```python
from build123d import *

# Parameters (mm, degrees)
SKETCH_1_W                  = 25
SKETCH_1_H                  = 62
EXTRUDE_1_DEPTH             = 10
PATTERN_LINEAR_1_COUNT      = 2
PATTERN_LINEAR_1_PITCH      = 16
PATTERN_LINEAR_1_COUNT_DIR2 = 2
PATTERN_LINEAR_1_PITCH_DIR2 = 52


with BuildPart() as part:
    # Sketch 1 → Extrude 1 (new body)
    with BuildSketch(Plane(origin=(0, 0, 0), x_dir=(0, 0, -1), z_dir=(1, 0, 0))):
        Rectangle(SKETCH_1_W, SKETCH_1_H)
    extrude(amount=EXTRUDE_1_DEPTH)

    # Sketch 2 → Cut-Revolve 1 (revolve, cut)
    with BuildSketch(Plane(origin=(0, 26, 0), x_dir=(1, 0, 0), z_dir=(0, 1, 0)), mode=Mode.PRIVATE) as cut_revolve_1_sk:
        Polygon((0, 8), (0, 10.5), (0.433, 10.067), (9.567, 10.067), (10, 10.5), (10, 8), align=None)
    cut_revolve_1 = revolve(cut_revolve_1_sk.sketch.rotate(Axis((10, 26, -8), (-1, 0, 0)), 180), axis=Axis((10, 26, -8), (-1, 0, 0)), mode=Mode.SUBTRACT)

    # Pattern Linear 1: Cut-Revolve 1 2 × 2
    with Locations(*[(0, -j * PATTERN_LINEAR_1_PITCH_DIR2, i * PATTERN_LINEAR_1_PITCH) for i in range(PATTERN_LINEAR_1_COUNT) for j in range(PATTERN_LINEAR_1_COUNT_DIR2) if (i, j) != (0, 0)]):
        add(cut_revolve_1, mode=Mode.SUBTRACT)

    # Sketch 4 → Cut-Revolve 2 (revolve, cut)
    with BuildSketch(Plane(origin=(0, 23, 0), x_dir=(1, 0, 0), z_dir=(0, 1, 0)), mode=Mode.PRIVATE) as cut_revolve_2_sk:
        Polygon((0, 0), (0, 3.8), (5.555555556, 3.8), (5.555555556, 3.5), (2.055555556, 3.5), (1.555555556, 3), (1.555555556, 1.5), (4.155555556, 1.5), (5.021580959, 0), align=None)
    revolve(cut_revolve_2_sk.sketch.rotate(Axis((5.021580959, 23, 0), (-1, 0, 0)), 180), axis=Axis((5.021580959, 23, 0), (-1, 0, 0)), mode=Mode.SUBTRACT)

    # Sketch 5 → Cut-Revolve 3 (revolve, cut)
    with BuildSketch(Plane(origin=(0, 0, 0), x_dir=(1, 0, 0), z_dir=(0, 1, 0)), mode=Mode.PRIVATE) as cut_revolve_3_sk:
        Polygon((0, 0), (0, 3.8), (5.555555556, 3.8), (5.555555556, 3.5), (2.055555556, 3.5), (1.555555556, 3), (1.555555556, 1.5), (4.155555556, 1.5), (5.021580959, 0), align=None)
    revolve(cut_revolve_3_sk.sketch.rotate(Axis((5.021580959, 0, 0), (-1, 0, 0)), 180), axis=Axis((5.021580959, 0, 0), (-1, 0, 0)), mode=Mode.SUBTRACT)

    # Sketch 6 → Cut-Revolve 4 (revolve, cut)
    with BuildSketch(Plane(origin=(0, -23, 0), x_dir=(1, 0, 0), z_dir=(0, 1, 0)), mode=Mode.PRIVATE) as cut_revolve_4_sk:
        Polygon((0, 0), (0, 3.8), (5.555555556, 3.8), (5.555555556, 3.5), (2.055555556, 3.5), (1.555555556, 3), (1.555555556, 1.5), (4.155555556, 1.5), (5.021580959, 0), align=None)
    revolve(cut_revolve_4_sk.sketch.rotate(Axis((5.021580959, -23, 0), (-1, 0, 0)), 180), axis=Axis((5.021580959, -23, 0), (-1, 0, 0)), mode=Mode.SUBTRACT)

    # Sketch 7 → Revolve 1 (revolve)
    with BuildSketch(Plane(origin=(0, 0, 0), x_dir=(1, 0, 0), z_dir=(0, 1, 0)), mode=Mode.PRIVATE) as revolve_1_sk:
        Polygon((10, 0), (10, 4), (21.6, 4), (22, 3.6), (22, 0), align=None)
    revolve(revolve_1_sk.sketch.rotate(Axis((22, 0, 0), (-1, 0, 0)), 180), axis=Axis((22, 0, 0), (-1, 0, 0)))

    # Sketch 8 → Revolve 2 (revolve)
    with BuildSketch(Plane(origin=(0, -23, 0), x_dir=(1, 0, 0), z_dir=(0, 1, 0)), mode=Mode.PRIVATE) as revolve_2_sk:
        Polygon((10, 0), (10, 5), (52.6, 5), (53, 4.6), (53, 0), align=None)
    revolve(revolve_2_sk.sketch.rotate(Axis((53, -23, 0), (-1, 0, 0)), 180), axis=Axis((53, -23, 0), (-1, 0, 0)))

    # Sketch 9 → Revolve 3 (revolve)
    with BuildSketch(Plane(origin=(0, 23, 0), x_dir=(1, 0, 0), z_dir=(0, 1, 0)), mode=Mode.PRIVATE) as revolve_3_sk:
        Polygon((10, 0), (10, 5), (52.6, 5), (53, 4.6), (53, 0), align=None)
    revolve(revolve_3_sk.sketch.rotate(Axis((53, 23, 0), (-1, 0, 0)), 180), axis=Axis((53, 23, 0), (-1, 0, 0)))


solid = part.part
```
Can you work these out from the model? Positions are in its coordinate system, mm. A direction names the side the tool comes from. Give positions to 0.01 mm unless a question says otherwise; leave off trailing zeros. Order: outer loops, then holes, each group sorted by start corner. A loop starts at its lowest first (then second) coordinate and runs counter-clockwise, first axis right, second up. Notation, with made-up numbers: (66.5, -36.75) - (78.5, -36.75) arc R22 ccw to (78.5, -13.75) - close; hole circle Ø3 at (33, 79.5). An arc over 180 degrees is marked (long way). Use a Markdown table: item, result. Add a question column.
Q1. If we section it at D-D on z = -7.75: Count the separate pieces of the cut face and the enclosed holes in it, plus the area to 3 significant figures.
Q2. Please list where these lines run through material, in increasing order: line 1 along Y through (x, z) = (12.5, 3.25); line 2 along Y through (x, z) = (1.1, 0); line 3 along Y through (x, z) = (18.5, 1.75).
Q3. On a 3-axis mill with a long thin cutter (end or side, diameter ignored), from which of +Z, -Z, +X, -X, +Y, -Y can I reach the whole of each face in a straight line? I mean faces 1 (the flat face through (53, 23, 0)), 2 (the flat face through (1.556, -24.3, 1.3)). Say none if no direction works.
Q4. If we section it at B-B on x = 28: Write out the boundary of the cut face in (y, z), plus the area to 3 significant figures.
Q5. If we section it at C-C on y = 15.5: Write out the boundary of the cut face in (x, z).
Q6. I'm going to push flat-ended pins straight in: pin 1 (3 mm diameter, centred on y = 24.5, z = 1, fed in from -X); pin 2 (6 mm diameter, centred on x = 18, y = 5, fed in from +Z); pin 3 (3 mm diameter, centred on y = -5, z = -4, fed in from +X). Where does each tip first touch, or does it pass through?
Q7. If we mould it in two halves opening along Y, with no side actions, what happens to faces 3 (the flat face through (53, -23, 0)), 4 (the flat face through (10, 0, 6))? For each: released by +Y, released by -Y, zero draft, split by the parting line, or undercut.
Q8. If we section it at A-A on z = 8: Write out the boundary of the cut face in (x, y).
Answers follow:
| question | item | result |
|---|---|---|
| 1 | separate pieces | 3 |
| 1 | enclosed holes | 0 |
| 1 | area | 537 mm^2 |
| 2 | line 1 | y = -26.8 to -19.2, -2.33 to 2.33, 19.2 to 26.8 |
| 2 | line 2 | y = -31 to -26.8, -19.2 to -3.8, 3.8 to 19.2, 26.8 to 31 |
| 2 | line 3 | y = -27.68 to -18.32, -3.6 to 3.6, 18.32 to 27.68 |
| 3 | face 1 | +Z, -Z, +X, +Y, -Y |
| 3 | face 2 | -X |
| 4 | outline | circle Ø10 at (-23, 0); circle Ø10 at (23, 0) |
| 4 | area | 157 mm^2 |
| 5 | outline | (0, -12.5) - (10, -12.5) - (10, 12.5) - (0, 12.5) - close |
| 6 | pin 1 | stops at x = 1.56 |
| 6 | pin 2 | stops at z = 3.46 |
| 6 | pin 3 | stops at x = 10 |
| 7 | face 3 | zero draft |
| 7 | face 4 | undercut |
| 8 | outline | (0, -31) - (10, -31) - (10, -28.5) - (9.57, -28.07) - (0.43, -28.07) - (0, -28.5) - close; (0, -23.5) - (0.43, -23.93) - (9.57, -23.93) - (10, -23.5) - (10, 23.5) - (9.57, 23.93) - (0.43, 23.93) - (0, 23.5) - close; (0, 28.5) - (0.43, 28.07) - (9.57, 28.07) - (10, 28.5) - (10, 31) - (0, 31) - close |
